from build123d import *

# Parameters (mm, degrees)
SKETCH1_W           = 16.23
SKETCH1_H           = 17
BOSS_EXTRUDE1_DEPTH = 2
SKETCH2_W           = 0.749
SKETCH2_H           = 17
BOSS_EXTRUDE2_DEPTH = 0.75
SKETCH3_W           = 0.75
SKETCH3_H           = 17
BOSS_EXTRUDE4_DEPTH = 0.75
CUT_EXTRUDE1_DEPTH  = 16.776621323
CUT_EXTRUDE3_DEPTH  = 0.5


with BuildPart() as part:
    # Sketch1 → Boss-Extrude1 (new body)
    with BuildSketch(Plane.XY):
        with Locations((2.412127937, -2.350261097)):
            Rectangle(SKETCH1_W, SKETCH1_H)
    extrude(amount=BOSS_EXTRUDE1_DEPTH)

    # Sketch2 → Boss-Extrude2 (add)
    with BuildSketch(Plane(origin=(10.527127937, 0, 0), x_dir=(0, 0, -1), z_dir=(1, 0, 0))):
        with Locations((-1.6255, -2.350261097)):
            Rectangle(SKETCH2_W, SKETCH2_H)
    extrude(amount=BOSS_EXTRUDE2_DEPTH)

    # Sketch3 → Boss-Extrude4 (add)
    with BuildSketch(Plane.ZY.offset(5.702872063)):
        with Locations((1.625, -2.350261097)):
            Rectangle(SKETCH3_W, SKETCH3_H)
    extrude(amount=BOSS_EXTRUDE4_DEPTH)

    # Sketch4 → Cut-Extrude1 (cut, through all)
    with BuildSketch(Plane(origin=(0, 0, 0), x_dir=(-1, 0, 0), z_dir=(0, 0, -1))):
        Polygon((-7.517127937, 2.653975471), (-3.402127937, 2.653975471), (-3.402127937, 4.253975471), (-1.422127937, 4.253975471), (-1.422127937, 2.653975471), (2.692872063, 2.653975471), (2.692872063, 1.128975471), (4.532872063, 1.128975471), (4.532872063, -2.931024529), (2.692872063, -2.931024529), (2.692872063, -4.456024529), (-7.517127937, -4.456024529), (-7.517127937, -2.931024529), (-9.357127937, -2.931024529), (-9.357127937, 1.128975471), (-7.517127937, 1.128975471), align=None)
    extrude(amount=-CUT_EXTRUDE1_DEPTH, mode=Mode.SUBTRACT)

    # Sketch6 → Cut-Extrude3 (cut)
    with BuildSketch(Plane(origin=(0, 0, 0), x_dir=(-1, 0, 0), z_dir=(0, 0, -1))):
        with BuildLine():
            Line((-5.412127937, -10.850261097), (0.587872063, -10.850261097))
            ThreePointArc((0.587872063, -10.850261097), (-2.412127937, -7.850261097), (-5.412127937, -10.850261097))
        make_face()
    extrude(amount=-CUT_EXTRUDE3_DEPTH, mode=Mode.SUBTRACT)


solid = part.part
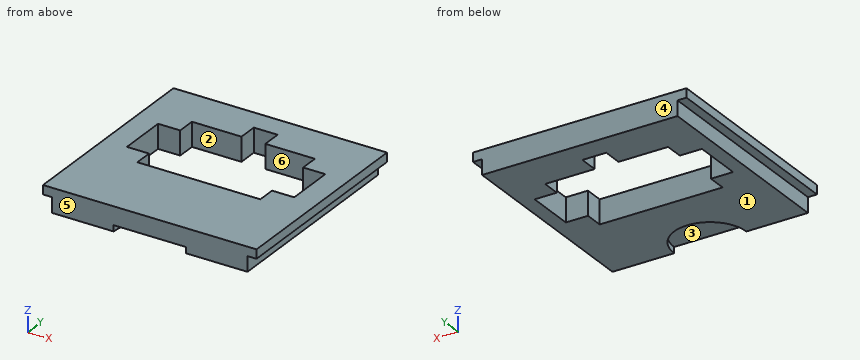
Source: CAD feature listing. Evaluate the final solid. Frame: model axes, mm. Face numbers are marked on the shaded views. A direction names the side the tool comes from. Round coordinates to 2 decimals unless told otherwise and drop trailing zeros. Order: outer loops, then holes, each group sorted by start corner. A loop starts at its lowest first (then second) coordinate and runs counter-clockwise, first axis right, second up. Notation, with made-up numbers: (74.25, -23.75) - (81.25, -23.75) arc R20 cw to (81.25, -15.75) - close; hole circle Ø3 at (27, 59.5). An arc over 180 degrees is marked (long way). Use a Markdown table: item, result. Add a question column.
1. Mould query, pull axis Y, two halves, no side actions, for the marked faces 4, 5 and 6. Classes: +Y half, -Y half, draft (parallel to the pull), parting line (faces both ways), or undercut.
2. Section query C-C (y = -0.5). Return the cut outline in (x, z).
3. Line query: probe 1 along X at (y, z) = (-2.5, 1.95); probe 2 along Y at (x, z) = (-2.25, 0.95); probe 3 along Y at (x, z) = (9, 1.3). Output: solid intervals per line, ascending.
4. Section query B-B (z = 0.3). Return the cut outline in (x, y).
5. Section query A-A (x = 9). Return the cut outline in (y, z).
6. First-contact query: pin 1 (0.6 mm diameter, centred on y = 0, z = 0.5, fed in from -X). Flat tip, straight axial feed; report the tip coordinate or a pass-through.
7. Set-up query: the marked faces 1, 2 and 3. Return all of +Z, -Z, +X, -X, +Y, -Y with unobstructed straight access to the full face (end or side cutting, diameter ignored); none if empty.
8. Section query D-D (y = -6.5). Return the cut outline in (x, z), then the cut area to 3 significant figures.
Derived:
| question | item | result |
|---|---|---|
| 1 | face 4 | +Y half |
| 1 | face 5 | -Y half |
| 1 | face 6 | undercut |
| 2 | outline | (-6.45, 1.25) - (-5.7, 1.25) - (-5.7, 0) - (-4.53, 0) - (-4.53, 2) - (-6.45, 2) - close; (9.36, 0) - (10.53, 0) - (10.53, 1.25) - (11.28, 1.25) - (11.28, 2) - (9.36, 2) - close |
| 3 | probe 1 | -6.45 to -4.53, 9.36 to 11.28 |
| 3 | probe 2 | -10.85 to -4.46, 2.65 to 6.15 |
| 3 | probe 3 | -10.85 to -2.93, 1.13 to 6.15 |
| 4 | outline | (-5.7, -10.85) - (-0.59, -10.85) arc R3 cw to (5.41, -10.85) - (10.53, -10.85) - (10.53, 6.15) - (-5.7, 6.15) - close; hole (-4.53, -2.93) - (-2.69, -2.93) - (-2.69, -4.46) - (7.52, -4.46) - (7.52, -2.93) - (9.36, -2.93) - (9.36, 1.13) - (7.52, 1.13) - (7.52, 2.65) - (3.4, 2.65) - (3.4, 4.25) - (1.42, 4.25) - (1.42, 2.65) - (-2.69, 2.65) - (-2.69, 1.13) - (-4.53, 1.13) - close |
| 5 | outline | (-10.85, 0) - (-2.93, 0) - (-2.93, 2) - (-10.85, 2) - close; (1.13, 0) - (6.15, 0) - (6.15, 2) - (1.13, 2) - close |
| 6 | pin 1 | x = -5.7 |
| 7 | face 1 | -Z, +X, -X, +Y, -Y |
| 7 | face 2 | +Z, -Z |
| 7 | face 3 | -Z, -Y |
| 8 | outline | (-6.45, 1.25) - (-5.7, 1.25) - (-5.7, 0) - (10.53, 0) - (10.53, 1.25) - (11.28, 1.25) - (11.28, 2) - (-6.45, 2) - close |
| 8 | area | 33.6 mm2 |
